Design review of the part built by this model. Coordinates are the model's own, in mm. Face numbers are marked on the shaded views. Coordinates: 2 decimals unless noted, no trailing zeros. Loops run counter-clockwise (first coordinate to the right, second up) from the corner with the lowest first, then second, coordinate; pieces in that order, holes last. Notation, with made-up numbers: (-5, -1.5) -> (10, -1.5) arc R32 cw to (10, 35.5) -> close; hole circle Ø8 at (-26, 10). An arc over 180 degrees is marked (long way). Use a Markdown table: item, result. Add a question column.
Q1. Draft analysis for pull direction Z (two halves, no side actions). For the marked faces 1, 2 and 3, state which applies: pulls with the +Z half, pulls with the -Z half, needs draft (parallel to the pull), parting line crosses it, or undercut.
Q2. Clearance check with a flat-ended pin moving along its axis: pin 1 Ø10 at (x, z) = (639.5, 211) entering from +Y. State where the tip first meets the part, or that it passes through.
Q3. For probe 1 along Y at (x, z) = (941, 237), list the stretches that pass through material, from the lowest coordinate up.
Q4. Take a section at A-A on x = 846.5. Write out the cut boundary in (y, z).
Q5. Take a section at B-B on z = 185. Write out the cut boundary in (x, y).
from build123d import *

# Parameters (mm, degrees)
F0_W     = 1000
F0_H     = 320
F1_DEPTH = 650
F2_W     = 1000
F2_H     = 120
F2_H_2   = 125
F3_DEPTH = 28
F4_DEPTH = 25
F5_W     = 1000
F5_H     = 6.141096
F6_DEPTH = 25


with BuildPart() as f1:
    # F0 (on Front) → F1 (new body)
    with BuildSketch(Plane.XZ):
        with Locations((500, 160)):
            Rectangle(F0_W, F0_H)
    extrude(amount=F1_DEPTH)

    # F2 (on face) → F3 (join)
    with BuildSketch(Plane(origin=(0, 0, 0), x_dir=(-1, 0, 0), z_dir=(0, 1, 0))):
        with Locations((-500, 220)):
            Rectangle(F2_W, F2_H)
        with Locations((-500, 62.5)):
            Rectangle(F2_W, F2_H_2)
    extrude(amount=-F3_DEPTH)

    # F2 (on face) → F4 (cut)
    with BuildSketch(Plane(origin=(0, 0, 0), x_dir=(-1, 0, 0), z_dir=(0, 1, 0))):
        with Locations((-500, 220)):
            Rectangle(F2_W, F2_H)
    extrude(amount=-F4_DEPTH, mode=Mode.SUBTRACT)

    # F5 (on face) → F6 (cut)
    with BuildSketch(Plane(origin=(0, 0, 0), x_dir=(-1, 0, 0), z_dir=(0, 1, 0))):
        with Locations((-500, 121.929452)):
            Rectangle(F5_W, F5_H)
    extrude(amount=-F6_DEPTH, mode=Mode.SUBTRACT)


solid = f1.part
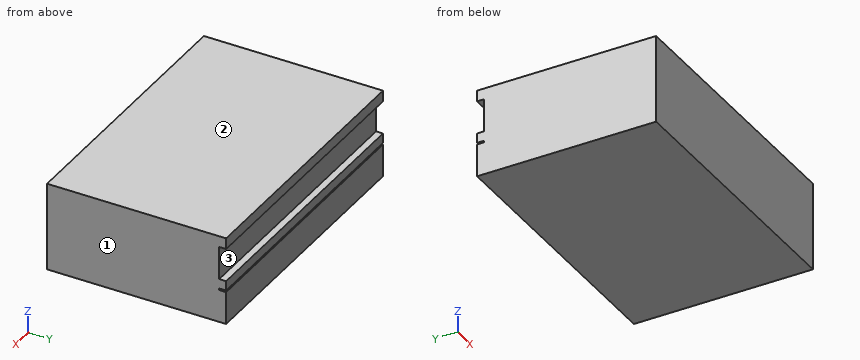
Answer list:
| question | item | result |
|---|---|---|
| 1 | face 1 | needs draft |
| 1 | face 2 | pulls with the +Z half |
| 1 | face 3 | undercut |
| 2 | pin 1 | y = -25 |
| 3 | probe 1 | -650 to -25 |
| 4 | outline | (-650, 0) -> (0, 0) -> (0, 118.86) -> (-25, 118.86) -> (-25, 125) -> (0, 125) -> (0, 160) -> (-25, 160) -> (-25, 280) -> (0, 280) -> (0, 320) -> (-650, 320) -> close |
| 5 | outline | (0, -650) -> (1000, -650) -> (1000, -25) -> (0, -25) -> close |
